from build123d import *

# Parameters (mm, degrees)
SKETCH1_R                = 1.815
BOSS_EXTRUDE1_DEPTH      = 0.4
BOSS_EXTRUDE2_DEPTH      = 4.835
BOSS_EXTRUDE2_DEPTH_BACK = 4.835


with BuildPart() as part:
    # Sketch1 → Boss-Extrude1 (new body)
    with BuildSketch(Plane.XY):
        with BuildLine():
            Line((-11.43, 0), (11.43, 0))
            Line((11.43, 0), (0.797330841, -14.046658294))
            ThreePointArc((0.797330841, -14.046658294), (0, -14.44311581), (-0.797330841, -14.046658294))
            Line((-0.797330841, -14.046658294), (-11.43, 0))
        make_face()
        with Locations((0, -5.82)):
            Circle(SKETCH1_R, mode=Mode.SUBTRACT)
    extrude(amount=BOSS_EXTRUDE1_DEPTH)

    # Sketch3 → Boss-Extrude2 (add, two sides)
    with BuildSketch(Plane(origin=(0, 0, 0), x_dir=(0, 0, -1), z_dir=(1, 0, 0))) as boss_extrude2_sk:
        with BuildLine():
            Line((-0.4, 0), (0, 0))
            Line((0, 0), (0, 3.718694726))
            ThreePointArc((0, 3.718694726), (-2.349771666, 4.332290684), (-0.6, 2.648180831))
            Line((-0.6, 2.648180831), (-0.6, 3.16914946))
            ThreePointArc((-0.6, 3.16914946), (-2.058445704, 4.011098557), (-0.4, 3.718694726))
            Line((-0.4, 3.718694726), (-0.4, 0))
        make_face()
    extrude(amount=BOSS_EXTRUDE2_DEPTH)
    extrude(boss_extrude2_sk.sketch, amount=-BOSS_EXTRUDE2_DEPTH_BACK)


solid = part.part
Geometry check sheet. Reference: the model listing, model coordinates, mm. A direction names the side the tool comes from. Round coordinates to 2 decimals unless told otherwise and drop trailing zeros. Write each loop counter-clockwise with the first axis right and the second up, starting at its lowest first coordinate (ties: lowest second). Pieces come first, ordered by that corner, then holes.
Item 1: Section check A-A (x = 0). Record the boundary of the cut face in (y, z) (3 decimals), plus the area to 3 significant figures.
Determined:
outline: (-14.443, 0) - (-7.635, 0) - (-7.635, 0.4) - (-14.443, 0.4) - close; (-4.005, 0) - (3.719, 0) arc R1.255 ccw (long way) to (2.648, 0.6) - (3.169, 0.6) arc R0.855 cw (long way) to (3.719, 0.4) - (-4.005, 0.4) - close
area: 8.09 mm2
Item 2: Mould release check, pull along Z, two halves, no side actions. Record for faces 1 (the face through (0.07, 3.98, 2.07)), 2 (the face through (0, -3, 0)), 3 (the face through (-1.44, -6.924, 0.197)): +Z half, -Z half, draft (parallel to the pull), parting line (faces both ways), or undercut.
Determined:
face 1: undercut
face 2: -Z half
face 3: draft
Item 3: Section check B-B (z = 0.9). Record the boundary of the cut face in (x, y) (3 decimals).
Determined:
outline: (-4.835, 2.515) - (4.835, 2.515) - (4.835, 2.941) - (-4.835, 2.941) - close; (-4.835, 4.497) - (4.835, 4.497) - (4.835, 4.922) - (-4.835, 4.922) - close
Item 4: Access from +Z, -Z, +X, -X, +Y, -Y to the whole of each face (thin tool, end or side, straight path). Record for faces 4 (the face through (-6.04, -7.12, 0.2)), 5 (the face through (4.835, 2.7, 1)), 6 (the face through (-4.835, 2.7, 1)).
Determined:
face 4: +Z, -Z, -X, -Y
face 5: +Z, -Z, +X, +Y
face 6: +Z, -Z, -X, +Y
Item 5: Go/stop test with a flat-tipped pin: pin 1 Ø9 at (x, y) = (-4, -5.5) entering from +Z. Record where the tip stops, or that it passes through.
Determined:
pin 1: stops at z = 0.4
Item 6: Material ranges on line 1 along Z through (x, y) = (1.5, -3); line 2 along Y through (x, z) = (0, 0.3) (3 decimals); line 3 along Y through (x, z) = (0, 0.2) (3 decimals), recorded low to high.
Determined:
line 1: z = 0 to 0.4
line 2: y = -14.443 to -7.635, -4.005 to 4.533
line 3: y = -14.443 to -7.635, -4.005 to 4.398
Item 7: Section check D-D (y = 1.5). Record the boundary of the cut face in (x, z) (3 decimals).
Determined:
outline: (-4.835, 0) - (4.835, 0) - (4.835, 0.4) - (-4.835, 0.4) - close
Item 8: Section check C-C (y = -5.82). Record the boundary of the cut face in (x, z) (3 decimals), plus the area to 3 significant figures.
Determined:
outline: (-7.025, 0) - (-1.815, 0) - (-1.815, 0.4) - (-7.025, 0.4) - close; (1.815, 0) - (7.025, 0) - (7.025, 0.4) - (1.815, 0.4) - close
area: 4.17 mm2
